Autodesk Inventor part; units mm, degrees
ref_plane "Work Plane1" through (46, 0, 25) normal (0.9659, 0, 0.2588) x (0, -1, 0)
ref_plane "Work Plane2" through (46, 0, 25) normal (0.8365, 0.5, 0.2241) x (0.2588, 0, -0.9659)
ref_plane "YZ Plane" through (0, 0, 0) normal (1, 0, 0) x (0, 1, 0)
sketch "Sketch1" plane through (0, 0, 0) normal (0, 0, 1) x (1, 0, 0)
  circle A0 centre (0, 0) radius 5
  circle A1 centre (0, 0) radius 8.45
  circle A2 centre (0, 0) radius 42.5
  circle A3 centre (0, 0) radius 45 construction
  circle A4 centre (-31.8198, 31.8198) radius 1.45
  arc A5 (-28.0933, 35.1535) -> (-35.1535, 28.0933) centre (-31.8198, 31.8198) ccw
  arc A6 (-35.1535, -28.0933) -> (-28.0933, -35.1535) centre (-31.8198, -31.8198) ccw
  circle A7 centre (-31.8198, -31.8198) radius 1.45
  arc A8 (28.0933, -35.1535) -> (35.1535, -28.0933) centre (31.8198, -31.8198) ccw
  circle A9 centre (31.8198, -31.8198) radius 1.45
  arc A10 (35.1535, 28.0933) -> (28.0933, 35.1535) centre (31.8198, 31.8198) ccw
  circle A11 centre (31.8198, 31.8198) radius 1.45
  line L0 (-31.8198, 31.8198) -> (31.8198, 31.8198) construction
  arc A12 (28.841, 35.8357) -> (-28.841, 35.8357) centre (0, 0) ccw
  arc A13 (-35.8357, 28.841) -> (-35.8357, -28.841) centre (0, 0) ccw
  arc A14 (-28.841, -35.8357) -> (28.841, -35.8357) centre (0, 0) ccw
  arc A15 (35.8357, -28.841) -> (35.8357, 28.841) centre (0, 0) ccw
  point P0 (0, -46)
  point P1 (0, 46)
  dimension "d0" = 10
  dimension "d1" = 16.9
  dimension "d2" = 85
  dimension "d3" = 90
  dimension "d4" = 2.9
  dimension "d5" = 5
  dimension "d8" = 360
  dimension "d25" = 92
extrude "Extrusion1" add sketch "Sketch1" along normal mid plane 7.5 contours A2
extrude "Extrusion3" add sketch "Sketch1" against normal blind 3.75 contours A12 A10 A15 A8 A14 A6 A13 A5
extrude "Extrusion4" add sketch "Sketch1" along normal blind 25 contours A12 A10 A15 A8 A14 A6 A13 A5
sketch "Sketch2" plane through (0, 0, 25) normal (0, 0, 1) x (1, 0, 0)
  arc A0 (35.8357, -28.841) -> (35.8357, 28.841) centre (0, 0) ccw construction
  line L0 (46, 0) -> (46, -31.8198) construction
  point P0 (31.8198, -31.8198)
ref_plane "Work Plane1" through (46, 0, 25) normal (0.9659, 0, 0.2588) x (0, -1, 0)
sketch "Sketch3" plane through (46, 0, 25) normal (0.9659, 0, 0.2588) x (0, -1, 0)
  line L0 (0, 0) -> (0, 12.2425) construction
ref_plane "Work Plane2" through (46, 0, 25) normal (0.8365, 0.5, 0.2241) x (0.2588, 0, -0.9659)
sketch "Sketch4" plane through (46, 0, 25) normal (0.8365, 0.5, 0.2241) x (0.2588, 0, -0.9659)
  circle A0 centre (0, 0) radius 5.325
  ellipse E0 centre (-11.9057, 22.2163) end of major axis (-17.5492, 64.3399) minor radius 9.5261
  line L0 (0, 0) -> (-0.9178, 0) construction
  point P0 (12.2425, 25.4515)
  point P1 (-0.4589, 0)
  dimension "d22" = 10.65
extrude "Extrusion5" cut sketch "Sketch4" along normal mid plane 25 contours A0 E0 | E0 A0 picked at (0.9978, 1.4954) picked at (-2.2508, 1.4196)
sketch "Sketch5" plane through (0, 0, -3.75) normal (0, 0, -1) x (-1, 0, 0)
  circle A0 centre (0, 0) radius 5
  circle A1 centre (0, 0) radius 8.45
extrude "Extrusion6" add sketch "Sketch5" against normal blind 2.5
properties part number "Case Part 1"
Source: CAD feature listing. Evaluate the final solid. Frame: model axes, mm. A direction names the side the tool comes from. Give positions to 0.01 mm unless a question says otherwise; leave off trailing zeros. Order: outer loops, then holes, each group sorted by start corner. A loop starts at its lowest first (then second) coordinate and runs counter-clockwise, first axis right, second up. Notation, with made-up numbers: (11.5, 34) -> (26.5, 34) arc R9 ccw to (26.5, 50) -> close; hole circle Ø4 at (-23.75, 24.25). An arc over 180 degrees is marked (long way). Use a Markdown table: item, result.
Q1. Material intervals for line 1 (Y direction, x = -33, z = 23); line 2 (X direction, y = 31, z = 21.25); line 3 (Z direction, x = 6.5, y = 30.5), sorted ascending. Write a range as [from, to].
A:
| item | result |
|---|---|
| line 1 | [-36.68, -32.66], [-30.98, -26.78], [26.78, 30.98], [32.66, 36.68] |
| line 2 | [-36.75, -33.02], [-30.62, -29.07], [29.07, 30.62], [33.02, 36.75] |
| line 3 | [-3.75, 3.75] |
Q2. Pull-direction query (Z, two-part tool) for faces 3 (the face through (44.753, -1.517, 19.153)), 4 (the face through (35.28, 35.43, 10.42)), 5 (the face through (1, -10, -3.75)); classes: +Z half, -Z half, draft (parallel to the pull), parting line (faces both ways), or undercut.
A:
| item | result |
|---|---|
| face 3 | undercut |
| face 4 | draft |
| face 5 | -Z half |
Q3. Section A-A (x = 0). Return the cut outline in (y, z).
A:
| item | result |
|---|---|
| outline | (-46, -3.75) -> (-5, -3.75) -> (-5, -1.25) -> (-8.45, -1.25) -> (-8.45, 3.75) -> (-42.5, 3.75) -> (-42.5, 25) -> (-46, 25) -> close; (5, -3.75) -> (46, -3.75) -> (46, 25) -> (42.5, 25) -> (42.5, 3.75) -> (8.45, 3.75) -> (8.45, -1.25) -> (5, -1.25) -> close |
Q4. Access query for faces 1 (the face through (0, 46, 10)), 2 (the face through (8.06, -2.54, 1.21)). Directions: +Z, -Z, +X, -X, +Y, -Y. A direction counts if a zero-diameter tool reaches every point of the face in a straight line with its end or side. Return the directions, or none.
A:
| item | result |
|---|---|
| face 1 | +Z, -Z, +Y |
| face 2 | +Z |
Q5. First-contact query: P1, Ø2.5, axis at x = -31.82, y = 31.82, coming from the -Z side; P2, Ø10, axis at y = 26.5, z = 20, coming from the -X side; P3, Ø5, axis at x = 15.5, z = 20, coming from the -Y side; P4, Ø4, axis at y = 26, z = 21, coming from the -X side. Flat tips, straight axial feed; report the tip coordinate or a pass-through.
A:
| item | result |
|---|---|
| P1 | through |
| P2 | x = -40.67 |
| P3 | y = -44.12 |
| P4 | x = -39.24 |
Q6. Section B-B (z = 6.25). Return the cut outline in (x, y), and give its area (3 significant figures).
A:
| item | result |
|---|---|
| outline | (-35.84, -28.84) arc R5 ccw to (-28.84, -35.84) arc R46 ccw to (28.84, -35.84) arc R5 ccw to (35.84, -28.84) arc R46 ccw to (35.84, 28.84) arc R5 ccw to (28.84, 35.84) arc R46 ccw to (-28.84, 35.84) arc R5 ccw to (-35.84, 28.84) arc R46 ccw to start; hole circle Ø85 at (0, 0); hole circle Ø2.9 at (-31.82, -31.82); hole circle Ø2.9 at (-31.82, 31.82); hole circle Ø2.9 at (31.82, -31.82); hole circle Ø2.9 at (31.82, 31.82) |
| area | 1,070 mm^2 |
Q7. Section D-D (x = 14). Return the cut outline in (y, z), and give its area (3 significant figures).
A:
| item | result |
|---|---|
| outline | (-43.82, -3.75) -> (43.82, -3.75) -> (43.82, 25) -> (40.13, 25) -> (40.13, 3.75) -> (-40.13, 3.75) -> (-40.13, 25) -> (-43.82, 25) -> close |
| area | 814 mm^2 |
Q8. Section C-C (y = 25.5). Return the cut outline in (x, z).
A:
| item | result |
|---|---|
| outline | (-38.29, -3.75) -> (38.29, -3.75) -> (38.29, 25) -> (34, 25) -> (34, 3.75) -> (-34, 3.75) -> (-34, 25) -> (-38.29, 25) -> close |
